For this review, take the finished solid that the model builds, in its own axes (mm). Face numbers are marked on the shaded views. A direction names the side the tool comes from. Round coordinates to 2 decimals unless told otherwise and drop trailing zeros. Write each loop counter-clockwise with the first axis right and the second up, starting at its lowest first coordinate (ties: lowest second). Pieces come first, ordered by that corner, then holes. Notation, with made-up numbers: (-2.75, 38) -> (31.25, 38) arc R37 ccw to (31.25, 77) -> close; hole circle Ø6 at (-12.75, 41). An arc over 180 degrees is marked (long way). Write item = value, one per line. Start each with the question number.
```python
from build123d import *

# Parameters (mm, degrees)
SKETCH_1_W      = 32
SKETCH_1_H      = 32
SKETCH_1_R      = 1.1
EXTRUDE_1_DEPTH = 1.4
SKETCH_2_W      = 18
SKETCH_2_H      = 18
EXTRUDE_2_DEPTH = 4
SKETCH_3_R      = 6.75
EXTRUDE_3_DEPTH = 12
SKETCH_5_W      = 4
SKETCH_5_H      = 9
EXTRUDE_4_DEPTH = 8
SKETCH_6_R      = 0.531026099
EXTRUDE_5_DEPTH = 4


with BuildPart() as part:
    # 草图1 → 凸台-拉伸1 (new body)
    with BuildSketch(Plane(origin=(0, 0, 0), x_dir=(1, 0, 0), z_dir=(0, 1, 0))):
        with Locations((16, 16)):
            Rectangle(SKETCH_1_W, SKETCH_1_H)
        with Locations(Location((3.25, 28.75, 0), (0, 0, 270))):
            Circle(SKETCH_1_R, mode=Mode.SUBTRACT)
        with Locations(Location((28.75, 28.75, 0), (0, 0, 90))):
            Circle(SKETCH_1_R, mode=Mode.SUBTRACT)
        with Locations(Location((28.75, 3.25, 0), (0, 0, 270))):
            Circle(SKETCH_1_R, mode=Mode.SUBTRACT)
        with Locations(Location((3.25, 3.25, 0), (0, 0, 90))):
            Circle(SKETCH_1_R, mode=Mode.SUBTRACT)
    extrude(amount=EXTRUDE_1_DEPTH)

    # 草图2 → 凸台-拉伸2 (add)
    with BuildSketch(Plane(origin=(0, 1.4, 0), x_dir=(1, 0, 0), z_dir=(0, 1, 0))):
        with Locations((16, 16)):
            Rectangle(SKETCH_2_W, SKETCH_2_H)
    extrude(amount=EXTRUDE_2_DEPTH)

    # 草图3 → 凸台-拉伸3 (add)
    with BuildSketch(Plane(origin=(0, 5.4, 0), x_dir=(1, 0, 0), z_dir=(0, 1, 0))):
        with Locations(Location((15.920011352, 16, 0), (0, 0, 270))):
            Circle(SKETCH_3_R)
    extrude(amount=EXTRUDE_3_DEPTH)

    # 草图4 → 切除-旋转1 (revolve, cut)
    with BuildSketch(Plane.XY.offset(-16), mode=Mode.PRIVATE) as cut_revolve_1_sk:
        Polygon((9.170011352, 11.4), (10.947526868, 9.4), (10.947526868, 5.4), (9.170011352, 5.4), align=None)
    revolve(cut_revolve_1_sk.sketch.rotate(Axis((15.920011352, 17.4, -16), (0, -1, 0)), 270), axis=Axis((15.920011352, 17.4, -16), (0, -1, 0)), mode=Mode.SUBTRACT)

    # 草图5 → 凸台-拉伸4 (add)
    with BuildSketch(Plane.XZ):
        with Locations((2.249894635, -23.15)):
            Rectangle(SKETCH_5_W, SKETCH_5_H)
    extrude(amount=EXTRUDE_4_DEPTH)

    # 草图6 → 凸台-拉伸5 (add)
    with BuildSketch(Plane.XZ.offset(8)):
        with Locations(Location((1.950545413, -20.513721841, 0), (0, 0, 90))):
            Circle(SKETCH_6_R)
        with Locations(Location((1.950545413, -22.513721841, 0), (0, 0, 90))):
            Circle(SKETCH_6_R)
        with Locations(Location((1.950545413, -24.513721841, 0), (0, 0, 90))):
            Circle(SKETCH_6_R)
        with Locations(Location((1.950545413, -26.513721841, 0), (0, 0, 90))):
            Circle(SKETCH_6_R)
    extrude(amount=EXTRUDE_5_DEPTH)


solid = part.part
```
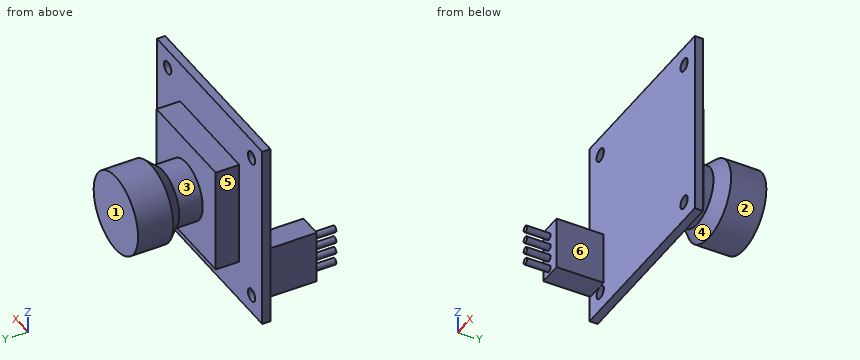
1. Draft analysis for pull direction Y (two halves, no side actions). For the marked faces 1, 2 and 3, state which applies: +Y half, -Y half, draft (parallel to the pull), parting line (faces both ways), or undercut.
2. Consider section A-A, the plane z = -28.75. Give the boundary of the cut face in (x, y), then the cut area to 3 significant figures.
3. Clearance check with flat-ended pins moving along their axes: pin 1 Ø2 at (x, y) = (14.5, 3) entering from -Z; pin 2 Ø2 at (x, y) = (24.5, 7) entering from +Z; pin 3 Ø2 at (x, y) = (14, 4) entering from +Z; pin 4 Ø3 at (y, z) = (4, -18.5) entering from +X. State where each tip first meets the part, or that it passes through.
4. Consider section C-C, the plane z = -16. Give the boundary of the cut face in (x, y).
5. Wall thickness on L1, parallel to X at y = 0.5, z = -28.75; L2, parallel to Z at x = 28, y = 0.25; L3, parallel to Y at x = 16.5, z = -9: over which ranges is each line inside the solid? List them lowest first. Write a range as from..to.
6. Consider section D-D, the plane x = 5. Give the boundary of the cut face in (y, z), then the cut area to 3 significant figures.
7. Machinability: for the marked faces 4, 5 and 6, which of the approach directions +Z, -Z, +X, -X, +Y, -Y give a long, thin tool a straight path to every point of the face, cutting with its end or side? Answer none if there is none.
8. Consider section B-B, the plane x = 28.75. Give the boundary of the cut face in (y, z).
Outcome:
q1.face_1 = +Y half
q1.face_2 = draft
q1.face_3 = undercut
q2.outline = (0, 0) -> (2.15, 0) -> (2.15, 1.4) -> (0, 1.4) -> close; (4.35, 0) -> (27.65, 0) -> (27.65, 1.4) -> (4.35, 1.4) -> close; (29.85, 0) -> (32, 0) -> (32, 1.4) -> (29.85, 1.4) -> close
q2.area = 38.6 mm2
q3.pin_1 = -25
q3.pin_2 = through
q3.pin_3 = -7
q3.pin_4 = 25
q4.outline = (0, 0) -> (32, 0) -> (32, 1.4) -> (25, 1.4) -> (25, 5.4) -> (20.89, 5.4) -> (20.89, 9.4) -> (22.67, 11.4) -> (22.67, 17.4) -> (9.17, 17.4) -> (9.17, 11.4) -> (10.95, 9.4) -> (10.95, 5.4) -> (7, 5.4) -> (7, 1.4) -> (0, 1.4) -> close
q5.L1 = 0..2.15, 4.35..27.65, 29.85..32
q5.L2 = -32..-29.55, -27.95..-4.05, -2.45..0
q5.L3 = 0..5.4
q6.outline = (0, -32) -> (1.4, -32) -> (1.4, 0) -> (0, 0) -> close
q6.area = 44.8 mm2
q7.face_4 = none
q7.face_5 = +Z, -Z, -X, +Y
q7.face_6 = +Z, -Z, +X, -Y
q8.outline = (0, -32) -> (1.4, -32) -> (1.4, -29.85) -> (0, -29.85) -> close; (0, -27.65) -> (1.4, -27.65) -> (1.4, -4.35) -> (0, -4.35) -> close; (0, -2.15) -> (1.4, -2.15) -> (1.4, 0) -> (0, 0) -> close
